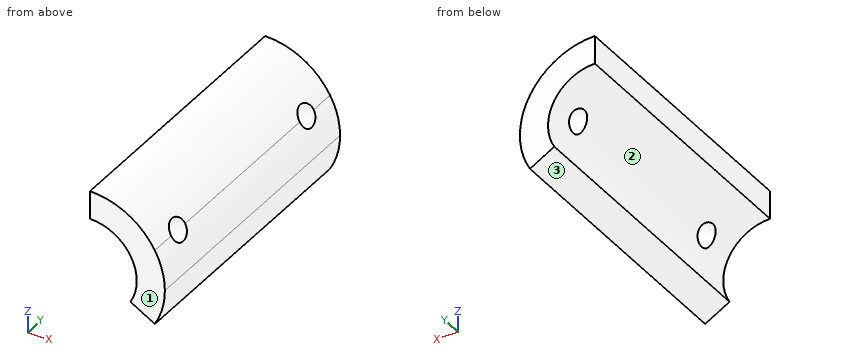
from build123d import *

# Parameters (mm, degrees)
F1_DEPTH = 75
F5_D     = 12


with BuildPart() as f1:
    # F0 (on Front) → F1 (new body, symmetric)
    with BuildSketch(Plane.XZ):
        with BuildLine():
            Line((21.6506350946, 12.5), (34.6410161514, 20))
            ThreePointArc((34.6410161514, 20), (20, 34.6410161514), (0, 40))
            Line((0, 40), (0, 25))
            ThreePointArc((0, 25), (12.5, 21.6506350946), (21.6506350946, 12.5))
        make_face()
        with BuildLine():
            ThreePointArc((34.6410161514, -20), (38.6370330516, -10.3527618041), (40, 0))
            ThreePointArc((40, 0), (38.6370330516, 10.3527618041), (34.6410161514, 20))
            Line((34.6410161514, 20), (21.6506350946, 12.5))
            ThreePointArc((21.6506350946, 12.5), (24.1481456572, 6.4704761276), (25, 0))
            ThreePointArc((25, 0), (24.1481456572, -6.4704761276), (21.6506350946, -12.5))
            Line((21.6506350946, -12.5), (34.6410161514, -20))
        make_face()
    extrude(amount=F1_DEPTH, both=True)

    # F5 (through all)
    with Locations(Plane(origin=(34.6410161514, 0, 20), x_dir=(0, -1, 0), z_dir=(0.8660254038, 0, 0.5))):
        with Locations((55, 0), (-55, 0)):
            Hole(F5_D / 2)


solid = f1.part
Build history of the part. All positions in model axes, mm. Face numbers are marked on the shaded views. Round coordinates to 2 decimals unless told otherwise and drop trailing zeros. Write each loop counter-clockwise with the first axis right and the second up, starting at its lowest first coordinate (ties: lowest second). Pieces come first, ordered by that corner, then holes. Notation, with made-up numbers: M 39,12.5 L 62,12.5 A22 ccw 62,32.5 Z; hole C -37.75,36 d6. An arc over 180 degrees is marked long. Answer as a JSON object with one key per item and string values. Group by question number.
(1) Mould opens along Z. For the marked faces 1, 2 and 3 say: pulls with the +Z half, pulls with the -Z half, needs draft (parallel to the pull), parting line crosses it, or undercut.
(2) Cut at D-D (x = 9). Give the cut face in (y, z), and give its area (3 significant figures).
(3) Cut at A-A (y = 58). Give the cut face in (x, z).
(4) Flat gauge pins, fed straight in: pin 1 (6 mm diameter, centred on x = 7.5, y = 2, fed in from +Z); pin 2 (1.5 mm diameter, centred on y = -58, z = 2, fed in from +X); pin 3 (10 mm diameter, centred on x = 15, z = 4.5, fed in from +Y); pin 4 (10 mm diameter, centred on y = 14, z = 17.5, fed in from -X). Where does each tip first touch, or does it go through?
(5) Cut at C-C (z = 15). Give the number of separate pieces and of enclosed holes in the cut face, and give its area (3 significant figures).
(6) Cut at B-B (y = -5.5). Give the cut face in (x, z), and give its area (3 significant figures).
(7) Drill centre lines: L1, parallel to X at y = 13, z = -3.5; L2, parallel to Z at x = 21, y = 21.5; L3, parallel to X at y = -9.5, z = 19.5. Where is each one in solid material? Low to high.
Responses:
{
 "1": {"face 1": "needs draft", "face 2": "undercut", "face 3": "pulls with the -Z half"},
 "2": {"outline": "M -75,23.32 L 75,23.32 L 75,38.97 L -75,38.97 Z", "area": "2,350 mm2"},
 "3": {"outline": "M 0,25 A25 cw 18.58,16.73 L 31.75,24.33 A40 ccw 0,40 Z; M 21.65,-12.5 L 34.64,-20 A40 ccw 36.95,15.33 L 23.78,7.73 A25 cw Z"},
 "4": {"pin 1": "stops at z = 39.75", "pin 2": "stops at x = 39.98", "pin 3": "passes through", "pin 4": "stops at x = 10.9"},
 "5": {"separate pieces": "3", "enclosed holes": "0", "area": "2,200 mm2"},
 "6": {"outline": "M 0,25 A25 cw 21.65,-12.5 L 34.64,-20 A40 ccw 0,40 Z", "area": "1,020 mm2"},
 "7": {"L1": "x = 24.75 to 39.85", "L2": "z = 13.56 to 34.04", "L3": "x = 15.64 to 34.92"}
}
